from build123d import *

# Parameters (mm, degrees)
F0_W     = 78.947164
F0_H     = 45.840274
F1_DEPTH = 12.7
F2_R     = 15
F2_R_2   = 10
F3_DEPTH = 25.4


with BuildPart() as f1:
    # F0 (on Front) → F1 (new body, symmetric)
    with BuildSketch(Plane.XZ):
        Rectangle(F0_W, F0_H)
    extrude(amount=F1_DEPTH, both=True)

    # F2 (on face) → F3 (join)
    with BuildSketch(Plane.XZ.offset(12.7)):
        Circle(F2_R)
        Circle(F2_R_2, mode=Mode.SUBTRACT)
    extrude(amount=F3_DEPTH)


solid = f1.part
CAD build for the part. Positions are in the model's coordinates, mm. A direction names the side the tool comes from. Round coordinates to 2 decimals unless told otherwise and drop trailing zeros. Order: outer loops, then holes, each group sorted by start corner. A loop starts at its lowest first (then second) coordinate and runs counter-clockwise, first axis right, second up. Notation, with made-up numbers: (-5.75, -12.75) -> (43.25, -12.75) arc R13 ccw to (43.25, 8.25) -> close; hole circle Ø4 at (33, 56). An arc over 180 degrees is marked (long way). Write item = value, one per line. Start each with the question number.
(1) Which spindle directions (+Z, -Z, +X, -X, +Y, -Y) get a long thin tool onto all of the face, cutting with end or side? Do faces 1 (the cylindrical face through (-14.985, -25.222, 0.66)), 2 (the flat face through (-1, 0, -22.92)). Say none if no direction does.
(2) Pull direction X, two halves, no side cores. Call faces 3 (the flat face through (0, -12.7, 0)), 4 (the flat face through (-1, -12.7, 16)), 5 (the flat face through (39.474, 0, 0)), 6 (the cylindrical face through (-2.17, -25.22, -9.76)): released by +X, released by -X, zero draft, split by the parting line, or undercut.
(3) Cut at D-D, the plane z = 0. List the corners of the cut face in (x, y), then the cut area to 3 significant figures.
(4) Probe line 1 (Z direction, x = 0, y = -21); line 2 (Y direction, x = -31, z = -14); line 3 (Z direction, x = 6, y = -28). List the from-to ranges inside material, lowest first. Write a range as [from, to].
(5) Cut at B-B, the plane z = -14. List the corners of the cut face in (x, y).
(6) Cut at A-A, the plane x = 0. List the corners of the cut face in (y, z).
(7) Cut at C-C, the plane y = -33. List the corners of the cut face in (x, z).
(8) Pin check, flat tips, straight feed: P1, Ø3, axis at y = -29, z = -14, coming from the -X side; P2, Ø6, axis at y = -21, z = 11.5, coming from the +X side; P3, Ø3, axis at y = -29, z = 11, coming from the +X side. Stop position of each tip, or through.
Model answer:
q1.face_1 = -Y
q1.face_2 = -Z, +X, -X, +Y, -Y
q2.face_3 = undercut
q2.face_4 = zero draft
q2.face_5 = released by +X
q2.face_6 = undercut
q3.outline = (-39.47, -12.7) -> (-15, -12.7) -> (-15, -38.1) -> (-10, -38.1) -> (-10, -12.7) -> (10, -12.7) -> (10, -38.1) -> (15, -38.1) -> (15, -12.7) -> (39.47, -12.7) -> (39.47, 12.7) -> (-39.47, 12.7) -> close
q3.area = 2,260 mm2
q4.line_1 = [-15, -10], [10, 15]
q4.line_2 = [-12.7, 12.7]
q4.line_3 = [-13.75, -8], [8, 13.75]
q5.outline = (-39.47, -12.7) -> (-5.39, -12.7) -> (-5.39, -38.1) -> (5.39, -38.1) -> (5.39, -12.7) -> (39.47, -12.7) -> (39.47, 12.7) -> (-39.47, 12.7) -> close
q6.outline = (-38.1, -15) -> (-12.7, -15) -> (-12.7, -22.92) -> (12.7, -22.92) -> (12.7, 22.92) -> (-12.7, 22.92) -> (-12.7, 15) -> (-38.1, 15) -> (-38.1, 10) -> (-12.7, 10) -> (-12.7, -10) -> (-38.1, -10) -> close
q7.outline = circle Ø30 at (0, 0); hole circle Ø20 at (0, 0)
q8.P1 = -8.29
q8.P2 = 12.36
q8.P3 = 11.61
